from build123d import *

# Parameters (mm, degrees)
SKETCH1_R                                      = 4
BOSS_EXTRUDE1_DEPTH                            = 3.175
F_6_CLEARANCE_HOLE1_D                          = 3.6576
F_6_CLEARANCE_HOLE1_DEPTH                      = 8
F_6_CLEARANCE_HOLE1_TIP                        = 1.0988539
CSK_FOR_6_FLAT_HEAD_MACHINE_SCREW2_D           = 3.6576
CSK_FOR_6_FLAT_HEAD_MACHINE_SCREW2_DEPTH       = 8
CSK_FOR_6_FLAT_HEAD_MACHINE_SCREW2_CSINK_D     = 7.0866
CSK_FOR_6_FLAT_HEAD_MACHINE_SCREW2_CSINK_ANGLE = 82
CSK_FOR_6_FLAT_HEAD_MACHINE_SCREW2_TIP         = 1.0988539


with BuildPart() as part:
    # Sketch1 → Boss-Extrude1 (new body)
    with BuildSketch(Plane.XY):
        with BuildLine():
            ThreePointArc((-36, 0), (0, -36), (36, 0))
            ThreePointArc((36, 0), (0, 36), (-36, 0))
        make_face()
        Circle(SKETCH1_R, mode=Mode.SUBTRACT)
    extrude(amount=BOSS_EXTRUDE1_DEPTH)

    # #6 Clearance Hole1
    with Locations(Plane(origin=(0, 0, 0), x_dir=(1, 0, 0), z_dir=(0, 0, -1))):
        with Locations((-11.853175458, 23.118447862), (24.728671999, -7.965750509), (11.853175458, -23.118447862), (-7.965750509, -24.728671999), (-23.118447862, -11.853175458), (-24.728671999, 7.965750509), (7.965750509, 24.728671999), (23.118447862, 11.853175458)):
            Hole(F_6_CLEARANCE_HOLE1_D / 2, depth=F_6_CLEARANCE_HOLE1_DEPTH)
            with Locations((0, 0, -(F_6_CLEARANCE_HOLE1_DEPTH + F_6_CLEARANCE_HOLE1_TIP / 2))):  # 118° drill point
                Cone(0, F_6_CLEARANCE_HOLE1_D / 2, F_6_CLEARANCE_HOLE1_TIP, mode=Mode.SUBTRACT)

    # CSK for #6 Flat Head Machine Screw2
    with Locations(Plane(origin=(0, 0, 3.175), x_dir=(-1, 0, 0), z_dir=(0, 0, 1))):
        with Locations((0, -18), (-18, 0), (0, 18), (18, 0), (0, -8), (-8, 0), (0, 8), (8, 0)):
            CounterSinkHole(CSK_FOR_6_FLAT_HEAD_MACHINE_SCREW2_D / 2, CSK_FOR_6_FLAT_HEAD_MACHINE_SCREW2_CSINK_D / 2, depth=CSK_FOR_6_FLAT_HEAD_MACHINE_SCREW2_DEPTH, counter_sink_angle=CSK_FOR_6_FLAT_HEAD_MACHINE_SCREW2_CSINK_ANGLE)
            with Locations((0, 0, -(CSK_FOR_6_FLAT_HEAD_MACHINE_SCREW2_DEPTH + CSK_FOR_6_FLAT_HEAD_MACHINE_SCREW2_TIP / 2))):  # 118° drill point
                Cone(0, CSK_FOR_6_FLAT_HEAD_MACHINE_SCREW2_D / 2, CSK_FOR_6_FLAT_HEAD_MACHINE_SCREW2_TIP, mode=Mode.SUBTRACT)


solid = part.part
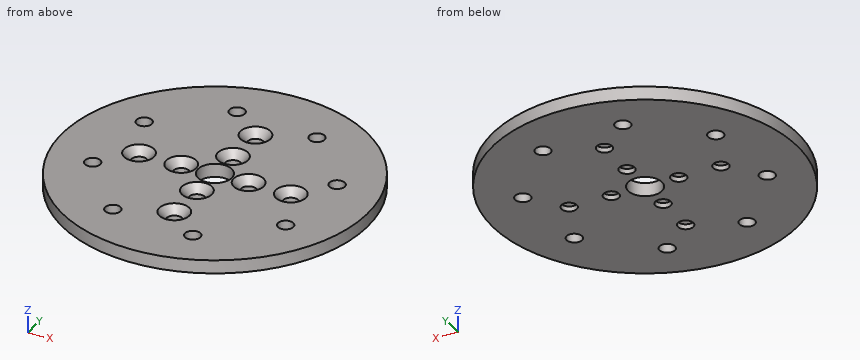
CAD build for the part. Positions are in the model's coordinates, mm. Coordinates: 2 decimals unless noted, no trailing zeros. Loops run counter-clockwise (first coordinate to the right, second up) from the corner with the lowest first, then second, coordinate; pieces in that order, holes last. Notation, with made-up numbers: (65, 88.25) - (106, 88.25) arc R25 ccw to (106, 104.25) - close; hole circle Ø1 at (7.5, -25). An arc over 180 degrees is marked (long way). Use one line per item in the form item = value. Start each with the question number.
1) Band-saw the part on D-D (x = -8). Give the cut face in (y, z) (3 decimals).
2) Flat gauge pins, fed straight in: pin 1 (5 mm diameter, centred on x = 0, y = 18, fed in from +Z); pin 2 (6 mm diameter, centred on x = -18, y = 0, fed in from +Z). Where does each tip first touch, or does it go through?
3) Band-saw the part on A-A (y = 18). Give the cut face in (x, z) (3 decimals).
4) Band-saw the part on C-C (z = 1.9). State how many separate pieces and enclosed holes the cut face has, and give its area (3 significant figures).
5) Drill centre lines: L1, parallel to Y at x = 0, z = 1.15; L2, parallel to X at y = -0.5, z = 0.4; L3, parallel to Y at x = 8.5, z = 1.6. Where is each one in solid material? Low to high. Write a range as from..to.
Check values:
q1.outline = (-35.1, 0) - (-1.829, 0) - (-1.829, 1.203) - (-3.543, 3.175) - (-35.1, 3.175) - close; (1.829, 0) - (22.9, 0) - (22.9, 3.175) - (3.543, 3.175) - (1.829, 1.203) - close; (26.557, 0) - (35.1, 0) - (35.1, 3.175) - (26.557, 3.175) - close
q2.pin_1 = 1.97
q2.pin_2 = 2.55
q3.outline = (-31.177, 0) - (-1.829, 0) - (-1.829, 1.203) - (-3.543, 3.175) - (-31.177, 3.175) - close; (1.829, 0) - (31.177, 0) - (31.177, 3.175) - (3.543, 3.175) - (1.829, 1.203) - close
q4.separate_pieces = 1
q4.enclosed_holes = 17
q4.area = 3,790 mm2
q5.L1 = -36..-19.83, -16.17..-9.83, -6.17..-4, 4..6.17, 9.83..16.17, 19.83..36
q5.L2 = -36..-19.76, -16.24..-9.76, -6.24..-3.97, 3.97..6.24, 9.76..16.24, 19.76..36
q5.L3 = -34.98..-26.48, -22.98..-2.12, 2.12..34.98
